Geometry: final body of the model. Coordinates: model frame, mm. A direction names the side the tool comes from. Round coordinates to 2 decimals unless told otherwise and drop trailing zeros. Write each loop counter-clockwise with the first axis right and the second up, starting at its lowest first coordinate (ties: lowest second). Pieces come first, ordered by that corner, then holes. Notation, with made-up numbers: M -21,69.5 L 0,69.5 A21 cw 0,106.5 Z; hole C 36,73.5 d3. An arc over 180 degrees is marked long. Answer as CSV lines item,"result". Start each with the question number.
Q1. Section query A-A on x = 322. Output: boundary loops of the cut face in (y, z).
Q2. Reachability of faces 4 (the flat face through (-812.8, 91, -4)), 5 (the flat face through (12, 91, 279.4)) from +Z, -Z, +X, -X, +Y, -Y: full face, straight path, thin tool, end or side. Return the list, or none.
Q3. Ray query, probe 1 along X at (y, z) = (171.5, -152); probe 2 along Z at (x, y) = (-147, 114.5); probe 3 along X at (y, z) = (160, -604). Return the intervals inside material, ascending.
Q4. Mould query, pull axis Z, two halves, no side actions, for faces 1 (the flat face through (-4, 184.15, -298)), 2 (the flat face through (-12, 91, -730.25)), 3 (the flat face through (-525, 91, -298.45)). Classes: pulls with the +Z half, pulls with the -Z half, needs draft (parallel to the pull), parting line crosses it, or undercut.
Q5. Section query B-B on z = -611.5. Output: boundary loops of the cut face in (x, y).
Q6. Section query C-C on y = 28. Output: boundary loops of the cut face in (x, z), and give its area (3 significant figures).
```python
from build123d import *

# Parameters (mm, degrees)
F0_W     = 787.4
F0_H     = 520.7
F0_W_2   = 819.15
F0_W_3   = 622.3
F0_H_2   = 450.85
F0_W_4   = 584.2
F0_H_3   = 196.85
F0_W_5   = 1041.4
F0_W_6   = 1003.3
F0_H_4   = 412.75
F1_DEPTH = 184.15


with BuildPart() as f1:
    # F0 (on Front) → F1 (new body)
    with BuildSketch(Plane.XZ):
        Polygon((831.85, -279.4), (831.85, 279.4), (-831.85, 279.4), (-831.85, -279.4), (-209.55, -279.4), align=None)
        with Locations((-419.1, 0)):
            Rectangle(F0_W, F0_H, mode=Mode.SUBTRACT)
        with Locations((403.225, 0)):
            Rectangle(F0_W_2, F0_H, mode=Mode.SUBTRACT)
        with Locations((-520.7, -504.825)):
            Rectangle(F0_W_3, F0_H_2)
        with Locations((-520.7, -612.775)):
            Rectangle(F0_W_4, F0_H_3, mode=Mode.SUBTRACT)
        with Locations((-520.7, -396.875)):
            Rectangle(F0_W_4, F0_H_3, mode=Mode.SUBTRACT)
        with Locations((311.15, -504.825)):
            Rectangle(F0_W_5, F0_H_2)
        with Locations((311.15, -504.825)):
            Rectangle(F0_W_6, F0_H_4, mode=Mode.SUBTRACT)
    extrude(amount=-F1_DEPTH)


solid = f1.part
```
Entries:
1,outline,"M 0,-730.25 L 184.15,-730.25 L 184.15,-711.2 L 0,-711.2 Z; M 0,-298.45 L 184.15,-298.45 L 184.15,-260.35 L 0,-260.35 Z; M 0,260.35 L 184.15,260.35 L 184.15,279.4 L 0,279.4 Z"
2,face 4,"+Y, -Y"
2,face 5,"+Z, +X, -X, +Y, -Y"
3,probe 1,"x = -831.85 to -812.8, -25.4 to -6.35, 812.8 to 831.85"
3,probe 2,"z = -730.25 to -711.2, -298.45 to -260.35, 260.35 to 279.4"
3,probe 3,"x = -831.85 to -812.8, -228.6 to -190.5, 812.8 to 831.85"
4,face 1,"needs draft"
4,face 2,"pulls with the -Z half"
4,face 3,"undercut"
5,outline,"M -831.85,0 L -812.8,0 L -812.8,184.15 L -831.85,184.15 Z; M -228.6,0 L -190.5,0 L -190.5,184.15 L -228.6,184.15 Z; M 812.8,0 L 831.85,0 L 831.85,184.15 L 812.8,184.15 Z"
6,outline,"M -831.85,-730.25 L 831.85,-730.25 L 831.85,279.4 L -831.85,279.4 Z; hole M -812.8,-711.2 L -228.6,-711.2 L -228.6,-514.35 L -812.8,-514.35 Z; hole M -812.8,-495.3 L -228.6,-495.3 L -228.6,-298.45 L -812.8,-298.45 Z; hole M -812.8,-260.35 L -25.4,-260.35 L -25.4,260.35 L -812.8,260.35 Z; hole M -190.5,-711.2 L 812.8,-711.2 L 812.8,-298.45 L -190.5,-298.45 Z; hole M -6.35,-260.35 L 812.8,-260.35 L 812.8,260.35 L -6.35,260.35 Z"
6,area,"199,000 mm^2"
